Design review of the part built by this model. Coordinates are the model's own, in mm. A direction names the side the tool comes from. Give positions to 0.01 mm unless a question says otherwise; leave off trailing zeros. Order: outer loops, then holes, each group sorted by start corner. A loop starts at its lowest first (then second) coordinate and runs counter-clockwise, first axis right, second up. Notation, with made-up numbers: (68, -12.75) -> (87, -12.75) arc R16 ccw to (87, 8.25) -> close; hole circle Ø4 at (47.25, 29.5). An arc over 180 degrees is marked (long way). Use a Markdown table: item, result. Add a question column.
```python
from build123d import *

# Parameters (mm, degrees)
F1_DEPTH = 12.7
F2_R     = 2.54


with BuildPart() as f1:
    # F0 (on Front) → F1 (new body)
    with BuildSketch(Plane.XZ):
        Polygon((-25.4, 0), (-25.4, -12.7), (-19.05, -12.7), (-19.05, -6.35), (19.05, -6.35), (19.05, -12.7), (25.4, -12.7), (25.4, 0), align=None)
    extrude(amount=-F1_DEPTH)

    # F2
    f2_edges = [f1.edges().sort_by_distance(p)[0] for p in [
        (-19.05, 6.35, -6.35),
        (19.05, 6.35, -6.35),
        (-25.4, 6.35, 0),
        (25.4, 6.35, 0),
    ]]
    fillet(f2_edges, radius=F2_R)


solid = f1.part
```
1) For L1, parallel to Z at x = -9, y = 7.75; L2, parallel to Z at x = 23, y = 1.25; L3, parallel to X at y = 8.5, z = -10.5, list the stretches that pass through material, from the lowest coordinate up. Write a range as [from, to].
2) Add section C-C (x = -12). Give the boundary of the cut face in (y, z), then the cut area to 3 significant figures.
3) Insertion check: pin 1 (4 mm diameter, centred on x = -0.5, z = -9.5, fed in from -Y); pin 2 (6.5 mm diameter, centred on x = 4.5, y = 6, fed in from -Z). Each pin has a flat end and moves straight along its axis. Give the tip position at first contact, or say it passes through.
4) Add section B-B (y = 9.75). Give the boundary of the cut face in (x, z), then the cut area to 3 significant figures.
5) The part is to be moulded in two halves that separate along X. For faces 1 (the cylindrical face through (24.676, 6.439, -0.764)), 2 (the flat face through (0, 6, 0)), 3 (the flat face through (19.05, 6, -11)), say which applies: +X half, -X half, draft (parallel to the pull), parting line (faces both ways), or undercut.
6) Machinability: for faces 4 (the cylindrical face through (18.286, 6.439, -7.074)), 5 (the flat face through (22, 6, -12.7)), which of the approach directions +Z, -Z, +X, -X, +Y, -Y give a long, thin tool a straight path to every point of the face, cutting with its end or side? Answer none if there is none.
7) Add section A-A (z = -9.75). Give the boundary of the cut face in (x, y), then the cut area to 3 significant figures.
Worked answers:
| question | item | result |
|---|---|---|
| 1 | L1 | [-6.35, 0] |
| 1 | L2 | [-12.7, 0] |
| 1 | L3 | [-25.4, -19.05], [19.05, 25.4] |
| 2 | outline | (0, -6.35) -> (12.7, -6.35) -> (12.7, 0) -> (0, 0) -> close |
| 2 | area | 80.6 mm^2 |
| 3 | pin 1 | through |
| 3 | pin 2 | z = -6.35 |
| 4 | outline | (-25.4, -12.7) -> (-19.05, -12.7) -> (-19.05, -8.89) arc R2.54 cw to (-16.51, -6.35) -> (16.51, -6.35) arc R2.54 cw to (19.05, -8.89) -> (19.05, -12.7) -> (25.4, -12.7) -> (25.4, -2.54) arc R2.54 ccw to (22.86, 0) -> (-22.86, 0) arc R2.54 ccw to (-25.4, -2.54) -> close |
| 4 | area | 403 mm^2 |
| 5 | face 1 | +X half |
| 5 | face 2 | draft |
| 5 | face 3 | undercut |
| 6 | face 4 | -Z, +Y, -Y |
| 6 | face 5 | -Z, +X, -X, +Y, -Y |
| 7 | outline | (-25.4, 0) -> (-19.05, 0) -> (-19.05, 12.7) -> (-25.4, 12.7) -> close; (19.05, 0) -> (25.4, 0) -> (25.4, 12.7) -> (19.05, 12.7) -> close |
| 7 | area | 161 mm^2 |
